Read the model definition and answer for the solid it produces. Units are mm, in the model's axes. A direction names the side the tool comes from. Give positions to 0.01 mm unless a question says otherwise; leave off trailing zeros. Order: outer loops, then holes, each group sorted by start corner. A loop starts at its lowest first (then second) coordinate and runs counter-clockwise, first axis right, second up. Notation, with made-up numbers: (52.25, -31) -> (63.25, -31) arc R14 ccw to (63.25, -12) -> close; hole circle Ø9 at (67, -1). An arc over 180 degrees is marked (long way). One line per item, written item: value. Start each with the question number.
from build123d import *

# Parameters (mm, degrees)
F0_W      = 90
F0_H      = 50
F1_DEPTH  = 2
F3_R      = 5.08
F4_R      = 5.08
F5_R      = 5.08
F6_R      = 5.08
F8_R      = 1.5
F9_DEPTH  = 25.4
F10_W     = 10
F10_H     = 4
F11_DEPTH = 25.4
F13_DEPTH = 25.4


with BuildPart() as f1:
    # F0 (on Top) → F1 (new body)
    with BuildSketch(Plane.XY):
        with Locations((45, 25)):
            Rectangle(F0_W, F0_H)
    extrude(amount=F1_DEPTH)

    # F3
    f3_edges = [f1.edges().sort_by_distance(p)[0] for p in [
        (90, 0, 1),
    ]]
    fillet(f3_edges, radius=F3_R)

    # F4
    f4_edges = [f1.edges().sort_by_distance(p)[0] for p in [
        (90, 50, 1),
    ]]
    fillet(f4_edges, radius=F4_R)

    # F5
    f5_edges = [f1.edges().sort_by_distance(p)[0] for p in [
        (0, 50, 1),
    ]]
    fillet(f5_edges, radius=F5_R)

    # F6
    f6_edges = [f1.edges().sort_by_distance(p)[0] for p in [
        (0, 0, 1),
    ]]
    fillet(f6_edges, radius=F6_R)

    # F8 (on offset) → F9 (cut)
    with BuildSketch(Plane.XY.offset(2)):
        with Locations((85, 5)):
            Circle(F8_R)
        with Locations((82.1494022449, 8.3385913854)):
            Circle(F8_R)
        with Locations((82.1494022449, 41.6614086146)):
            Circle(F8_R)
        with Locations((85, 45)):
            Circle(F8_R)
        with Locations((7.8505977551, 41.6614086146)):
            Circle(F8_R)
        with Locations((5, 45)):
            Circle(F8_R)
        with Locations((7.8505977551, 8.3385913854)):
            Circle(F8_R)
        with Locations((5, 5)):
            Circle(F8_R)
    extrude(amount=-F9_DEPTH, mode=Mode.SUBTRACT)

    # F10 (on offset) → F11 (cut)
    with BuildSketch(Plane.XY.offset(2)):
        with BuildLine():
            Line((35, 22.5), (35, 27.5))
            Line((35, 27.5), (35.8850657517, 27.5))
            add(Edge.make_bspline(
                [(35.8850657517, 27.5), (29.9931568267, 28.0368228686), (29.9931568267, 25)],
                knots=[4.5346839474, 4.5346839474, 4.5346839474, 6.2831853072, 6.2831853072, 6.2831853072], degree=2, weights=[1, 0.6415718139, 1]))
            add(Edge.make_bspline(
                [(29.9931568267, 25), (29.9931568267, 21.9631771314), (35.8850657517, 22.5)],
                knots=[0, 0, 0, 1.7485013598, 1.7485013598, 1.7485013598], degree=2, weights=[1, 0.6415718139, 1]))
            Line((35.8850657517, 22.5), (35, 22.5))
        make_face()
        with BuildLine():
            Line((35.8850657517, 27.5), (35, 27.5))
            Line((35, 27.5), (35, 22.5))
            Line((35, 22.5), (35.8850657517, 22.5))
            add(Edge.make_bspline(
                [(35.8850657517, 22.5), (40.0068431733, 22.8755428686), (40.0068431733, 25), (40.0068431733, 27.1244571314), (35.8850657517, 27.5)],
                knots=[1.7485013598, 1.7485013598, 1.7485013598, 3.1415926536, 3.1415926536, 4.5346839474, 4.5346839474, 4.5346839474], degree=2, weights=[1, 0.767062975, 1, 0.767062975, 1]))
        make_face()
        with BuildLine():
            Line((50, 27.5), (35.8850657517, 27.5))
            add(Edge.make_bspline(
                [(35.8850657517, 22.5), (40.0068431733, 22.8755428686), (40.0068431733, 25), (40.0068431733, 27.1244571314), (35.8850657517, 27.5)],
                knots=[1.7485013598, 1.7485013598, 1.7485013598, 3.1415926536, 3.1415926536, 4.5346839474, 4.5346839474, 4.5346839474], degree=2, weights=[1, 0.767062975, 1, 0.767062975, 1]))
            Line((35.8850657517, 22.5), (50, 22.5))
            Line((50, 22.5), (50, 27.5))
        make_face()
        with Locations((45, 30.5)):
            Rectangle(F10_W, F10_H)
        Polygon((40, 28.5), (40, 32.5), (35, 28.5), align=None)
        Polygon((35, 21.5), (40, 17.5), (40, 21.5), align=None)
        with Locations((45, 19.5)):
            Rectangle(F10_W, F10_H)
        with BuildLine():
            Line((58.6482731998, 30.5), (53, 32.5))
            ThreePointArc((53, 32.5), (51.4781820371, 30.5), (53, 28.5))
            Line((53, 28.5), (58.6482731998, 30.5))
        make_face()
        with BuildLine():
            ThreePointArc((53, 21.5), (51.4781820371, 19.5), (53, 17.5))
            Line((53, 17.5), (58.6482731998, 19.5))
            Line((58.6482731998, 19.5), (53, 21.5))
        make_face()
    extrude(amount=-F11_DEPTH, mode=Mode.SUBTRACT)

    # F12 (on offset) → F13 (cut)
    with BuildSketch(Plane.XY.offset(2)):
        Polygon((75.8748404465, 23.8996903335), (50.8748404465, 8.8996903335), (75.8748404465, 8.8996903335), align=None)
        Polygon((50.8748404465, 41.1003096665), (75.8748404465, 26.1003096665), (75.8748404465, 41.1003096665), align=None)
        Polygon((14.1251595535, 26.1003096665), (39.1251595535, 41.1003096665), (14.1251595535, 41.1003096665), align=None)
        Polygon((39.1251595535, 8.8996903335), (14.1251595535, 23.8996903335), (14.1251595535, 8.8996903335), align=None)
    extrude(amount=-F13_DEPTH, mode=Mode.SUBTRACT)


solid = f1.part
Item 1: Find section B-B on x = 19. Write down the section's boundary in (y, z).
Item 2: Find section C-C on x = 37. Write down the section's boundary in (y, z).
Item 3: Find section A-A on y = 37. Write down the section's boundary in (x, z), then the cut area to 3 significant figures.
Item 4: A tool of negligible diameter and unlimited length cuts with its end or side. For faces 1 (the flat face through (43, 27.5, 1)), 2 (the flat face through (0, 25, 1)), from which of +Z, -Z, +X, -X, +Y, -Y can it reach the whole face along a straight path? Write none if from no direction.
Item 5: For a pull along Y with two mould halves and no side action, classify faces 3 (the flat face through (90, 25, 1)), 4 (the flat face through (55.785, 29.486, 1.014)), 5 (the cylindrical face through (88.472, 1.449, 1.014)) as +Y half, -Y half, draft (parallel to the pull), parting line (faces both ways), or undercut.
Item 6: Find the intervals of material crossed by line 1 (Y direction, x = 85, z = 0.5); line 2 (Y direction, x = 45.5, z = 0.1); line 3 (X direction, y = 28, z = 0.8), in increasing order. Write a range as from..to.
Item 7: Find section D-D on z = 1.3. Count the separate pieces of the cut face and the enclosed holes in it, then the cut area to 3 significant figures.
Checks:
1. outline: (0, 0) -> (8.9, 0) -> (8.9, 2) -> (0, 2) -> close; (20.97, 0) -> (29.03, 0) -> (29.03, 2) -> (20.97, 2) -> close; (41.1, 0) -> (50, 0) -> (50, 2) -> (41.1, 2) -> close
2. outline: (0, 0) -> (8.9, 0) -> (8.9, 2) -> (0, 2) -> close; (10.17, 0) -> (19.9, 0) -> (19.9, 2) -> (10.17, 2) -> close; (21.5, 0) -> (22.5, 0) -> (22.5, 2) -> (21.5, 2) -> close; (27.5, 0) -> (28.5, 0) -> (28.5, 2) -> (27.5, 2) -> close; (30.1, 0) -> (39.83, 0) -> (39.83, 2) -> (30.1, 2) -> close; (41.1, 0) -> (50, 0) -> (50, 2) -> (41.1, 2) -> close
3. outline: (0, 0) -> (14.13, 0) -> (14.13, 2) -> (0, 2) -> close; (32.29, 0) -> (57.71, 0) -> (57.71, 2) -> (32.29, 2) -> close; (75.87, 0) -> (90, 0) -> (90, 2) -> (75.87, 2) -> close
3. area: 107 mm2
4. face 1: +Z, -Z
4. face 2: +Z, -Z, -X, +Y, -Y
5. face 3: draft
5. face 4: undercut
5. face 5: -Y half
6. line 1: 0..3.5, 6.5..43.5, 46.5..50
6. line 2: 0..17.5, 21.5..22.5, 27.5..28.5, 32.5..50
6. line 3: 0..14.13, 17.29..72.71, 75.87..90
7. separate pieces: 1
7. enclosed holes: 17
7. area: 3,440 mm2
